Source: CAD feature listing. Evaluate the final solid. Frame: model axes, mm. Round coordinates to 2 decimals unless told otherwise and drop trailing zeros. Answer in a Markdown table with one row per item. Add a question column.
Item 1: Cut plane A-A on z = 646. Give the number of separate pieces and of enclosed holes in the cut face, and give its area (3 significant figures).
Item 2: Contact query for flat-ended pins moving along their axis: pin 1 (1.5 mm diameter, centred on y = 1.5, z = 540, fed in from -X); pin 2 (8 mm diameter, centred on y = -3, z = 688.5, fed in from -X); pin 3 (0.6 mm diameter, centred on y = -18, z = 282, fed in from +X); pin 4 (0.9 mm diameter, centred on y = 3.5, z = 631, fed in from +X). Output: stop coordinate, or through.
Item 3: Material intervals for probe 1 along X at (y, z) = (13.5, 697); probe 2 along X at (y, z) = (15, 284); probe 3 along Y at (x, z) = (6.5, 113), sorted ascending.
from build123d import *

# Parameters (mm, degrees)
EXTRUDE1_DEPTH = 1020


with BuildPart() as part:
    # Sketch1 → Extrude1 (new body)
    with BuildSketch(Plane.XY):
        with BuildLine():
            Line((5.8, -20), (17, -20))
            ThreePointArc((17, -20), (19.121320344, -19.121320344), (20, -17))
            Line((20, -17), (20, -5.8))
            Line((20, -5.8), (18.5, -5.8))
            Line((18.5, -5.8), (18.5, -5))
            Line((18.5, -5), (14, -5))
            Line((14, -5), (14, -10.05))
            Line((14, -10.05), (11.464213562, -10.05))
            Line((11.464213562, -10.05), (7.5, -6.085786438))
            Line((7.5, -6.085786438), (7.5, 6.085786438))
            Line((7.5, 6.085786438), (11.464213562, 10.05))
            Line((11.464213562, 10.05), (14, 10.05))
            Line((14, 10.05), (14, 5))
            Line((14, 5), (18.5, 5))
            Line((18.5, 5), (18.5, 5.8))
            Line((18.5, 5.8), (20, 5.8))
            Line((20, 5.8), (20, 17))
            ThreePointArc((20, 17), (19.121320344, 19.121320344), (17, 20))
            Line((17, 20), (5.8, 20))
            Line((5.8, 20), (5.8, 18.5))
            Line((5.8, 18.5), (5, 18.5))
            Line((5, 18.5), (5, 14))
            Line((5, 14), (10.05, 14))
            Line((10.05, 14), (10.05, 11.464213562))
            Line((10.05, 11.464213562), (6.085786438, 7.5))
            Line((6.085786438, 7.5), (-6.085786438, 7.5))
            Line((-6.085786438, 7.5), (-10.05, 11.464213562))
            Line((-10.05, 11.464213562), (-10.05, 14))
            Line((-10.05, 14), (-5, 14))
            Line((-5, 14), (-5, 18.5))
            Line((-5, 18.5), (-5.8, 18.5))
            Line((-5.8, 18.5), (-5.8, 20))
            Line((-5.8, 20), (-17, 20))
            ThreePointArc((-17, 20), (-19.121320344, 19.121320344), (-20, 17))
            Line((-20, 17), (-20, 5.8))
            Line((-20, 5.8), (-18.5, 5.8))
            Line((-18.5, 5.8), (-18.5, 5))
            Line((-18.5, 5), (-14, 5))
            Line((-14, 5), (-14, 10.05))
            Line((-14, 10.05), (-11.464213562, 10.05))
            Line((-11.464213562, 10.05), (-7.5, 6.085786438))
            Line((-7.5, 6.085786438), (-7.5, -6.085786438))
            Line((-7.5, -6.085786438), (-11.464213562, -10.05))
            Line((-11.464213562, -10.05), (-14, -10.05))
            Line((-14, -10.05), (-14, -5))
            Line((-14, -5), (-18.5, -5))
            Line((-18.5, -5), (-18.5, -5.8))
            Line((-18.5, -5.8), (-20, -5.8))
            Line((-20, -5.8), (-20, -17))
            ThreePointArc((-20, -17), (-19.121320344, -19.121320344), (-17, -20))
            Line((-17, -20), (-5.8, -20))
            Line((-5.8, -20), (-5.8, -18.5))
            Line((-5.8, -18.5), (-5, -18.5))
            Line((-5, -18.5), (-5, -14))
            Line((-5, -14), (-10.05, -14))
            Line((-10.05, -14), (-10.05, -11.464213562))
            Line((-10.05, -11.464213562), (-6.085786438, -7.5))
            Line((-6.085786438, -7.5), (6.085786438, -7.5))
            Line((6.085786438, -7.5), (10.05, -11.464213562))
            Line((10.05, -11.464213562), (10.05, -14))
            Line((10.05, -14), (5, -14))
            Line((5, -14), (5, -18.5))
            Line((5, -18.5), (5.8, -18.5))
            Line((5.8, -18.5), (5.8, -20))
        make_face()
        with BuildLine():
            Line((14.5, -18.5), (9.5, -18.5))
            ThreePointArc((9.5, -18.5), (8, -17), (9.5, -15.5))
            Line((9.5, -15.5), (11.75, -15.5))
            Line((11.75, -15.5), (11.75, -14.5))
            ThreePointArc((11.75, -14.5), (12.555456352, -12.555456352), (14.5, -11.75))
            Line((14.5, -11.75), (15.5, -11.75))
            Line((15.5, -11.75), (15.5, -9.5))
            ThreePointArc((15.5, -9.5), (17, -8), (18.5, -9.5))
            Line((18.5, -9.5), (18.5, -14.5))
            Line((18.5, -14.5), (17.25, -14.5))
            ThreePointArc((17.25, -14.5), (16.444543648, -16.444543648), (14.5, -17.25))
            Line((14.5, -17.25), (14.5, -18.5))
        make_face(mode=Mode.SUBTRACT)
        with BuildLine():
            Line((18.5, 14.5), (17.25, 14.5))
            ThreePointArc((17.25, 14.5), (16.444543648, 16.444543648), (14.5, 17.25))
            Line((14.5, 17.25), (14.5, 18.5))
            Line((14.5, 18.5), (9.5, 18.5))
            ThreePointArc((9.5, 18.5), (8, 17), (9.5, 15.5))
            Line((9.5, 15.5), (11.75, 15.5))
            Line((11.75, 15.5), (11.75, 14.5))
            ThreePointArc((11.75, 14.5), (12.555456352, 12.555456352), (14.5, 11.75))
            Line((14.5, 11.75), (15.5, 11.75))
            Line((15.5, 11.75), (15.5, 9.5))
            ThreePointArc((15.5, 9.5), (17, 8), (18.5, 9.5))
            Line((18.5, 9.5), (18.5, 14.5))
        make_face(mode=Mode.SUBTRACT)
        with BuildLine():
            Line((5.5, 5.5), (2.397915762, 5.5))
            Line((2.397915762, 5.5), (1.998263135, 4.583333333))
            ThreePointArc((1.998263135, 4.583333333), (0, 5), (-1.998263135, 4.583333333))
            Line((-1.998263135, 4.583333333), (-2.397915762, 5.5))
            Line((-2.397915762, 5.5), (-5.5, 5.5))
            Line((-5.5, 5.5), (-5.5, 2.397915762))
            Line((-5.5, 2.397915762), (-4.583333333, 1.998263135))
            ThreePointArc((-4.583333333, 1.998263135), (-5, 0), (-4.583333333, -1.998263135))
            Line((-4.583333333, -1.998263135), (-5.5, -2.397915762))
            Line((-5.5, -2.397915762), (-5.5, -5.5))
            Line((-5.5, -5.5), (-2.397915762, -5.5))
            Line((-2.397915762, -5.5), (-1.998263135, -4.583333333))
            ThreePointArc((-1.998263135, -4.583333333), (0, -5), (1.998263135, -4.583333333))
            Line((1.998263135, -4.583333333), (2.397915762, -5.5))
            Line((2.397915762, -5.5), (5.5, -5.5))
            Line((5.5, -5.5), (5.5, -2.397915762))
            Line((5.5, -2.397915762), (4.583333333, -1.998263135))
            ThreePointArc((4.583333333, -1.998263135), (5, 0), (4.583333333, 1.998263135))
            Line((4.583333333, 1.998263135), (5.5, 2.397915762))
            Line((5.5, 2.397915762), (5.5, 5.5))
        make_face(mode=Mode.SUBTRACT)
        with BuildLine():
            Line((-18.5, -14.5), (-17.25, -14.5))
            ThreePointArc((-17.25, -14.5), (-16.444543648, -16.444543648), (-14.5, -17.25))
            Line((-14.5, -17.25), (-14.5, -18.5))
            Line((-14.5, -18.5), (-9.5, -18.5))
            ThreePointArc((-9.5, -18.5), (-8, -17), (-9.5, -15.5))
            Line((-9.5, -15.5), (-11.75, -15.5))
            Line((-11.75, -15.5), (-11.75, -14.5))
            ThreePointArc((-11.75, -14.5), (-12.555456352, -12.555456352), (-14.5, -11.75))
            Line((-14.5, -11.75), (-15.5, -11.75))
            Line((-15.5, -11.75), (-15.5, -9.5))
            ThreePointArc((-15.5, -9.5), (-17, -8), (-18.5, -9.5))
            Line((-18.5, -9.5), (-18.5, -14.5))
        make_face(mode=Mode.SUBTRACT)
        with BuildLine():
            Line((-14.5, 18.5), (-9.5, 18.5))
            ThreePointArc((-9.5, 18.5), (-8, 17), (-9.5, 15.5))
            Line((-9.5, 15.5), (-11.75, 15.5))
            Line((-11.75, 15.5), (-11.75, 14.5))
            ThreePointArc((-11.75, 14.5), (-12.555456352, 12.555456352), (-14.5, 11.75))
            Line((-14.5, 11.75), (-15.5, 11.75))
            Line((-15.5, 11.75), (-15.5, 9.5))
            ThreePointArc((-15.5, 9.5), (-17, 8), (-18.5, 9.5))
            Line((-18.5, 9.5), (-18.5, 14.5))
            Line((-18.5, 14.5), (-17.25, 14.5))
            ThreePointArc((-17.25, 14.5), (-16.444543648, 16.444543648), (-14.5, 17.25))
            Line((-14.5, 17.25), (-14.5, 18.5))
        make_face(mode=Mode.SUBTRACT)
    extrude(amount=EXTRUDE1_DEPTH)


solid = part.part
Results below:
| question | item | result |
|---|---|---|
| 1 | separate pieces | 1 |
| 1 | enclosed holes | 5 |
| 1 | area | 556 mm2 |
| 2 | pin 1 | x = -7.5 |
| 2 | pin 2 | x = -20 |
| 2 | pin 3 | x = 19.92 |
| 2 | pin 4 | x = 7.5 |
| 3 | probe 1 | -20 to -18.5, -11.94 to -10.05, 10.05 to 11.94, 18.5 to 20 |
| 3 | probe 2 | -20 to -17.2, -11.75 to -5, 5 to 11.75, 17.2 to 20 |
| 3 | probe 3 | -20 to -14, -7.91 to 7.91, 14 to 20 |
